```python
from build123d import *

# Parameters (mm, degrees)
F0_R     = 3.302
F0_R_2   = 16.51
F0_W     = 177.8
F0_H     = 77.7875
F1_DEPTH = 3.175


# Not quite as in the source:
# - ends of sketch curves that miss each other by under 0.0002 mm in the source are joined


with BuildPart() as f1:
    # F0 (on Front) → F1 (new body)
    with BuildSketch(Plane.XZ):
        with BuildLine():
            Line((-4.6405893252, -64.494198626), (72.172606051, -64.494198626))
            ThreePointArc((72.172606051, -64.494198626), (89.5045003647, -57.3150929397), (96.683606051, -39.983198626))
            Line((96.683606051, -39.983198626), (96.683606051, -30.0584486086))
            Line((96.683606051, -30.0584486086), (44.4719158113, 81.3992435336))
            Line((44.4719158113, 81.3992435336), (-29.9480052508, 81.3992435336))
            Line((-29.9480052508, 81.3992435336), (-35.9978974571, 50.6829957967))
            Line((-35.9978974571, 50.6829957967), (-19.4879078689, 50.6714224456))
            ThreePointArc((-19.4879078689, 50.6714224456), (-15.5812211009, 47.1637298884), (-13.9720730804, 42.1660573792))
            Line((-13.9720730804, 42.1660573792), (-5.4024819992, 38.3506346508))
            Line((-5.4024819992, 38.3506346508), (-2.9009456417, 36.1038269705))
            Line((-2.9009456417, 36.1038269705), (-2.3647786124, 27.9011076368))
            ThreePointArc((-2.3647786124, 27.9011076368), (3.4353485173, 23.5426794776), (4.3712937617, 16.3481414632))
            Line((4.3712937617, 16.3481414632), (4.2880776677, 1.0115236557))
            Line((4.2880776677, 1.0115236557), (-4.6405893252, -15.5276898319))
            Line((-4.6405893252, -15.5276898319), (-105.627393949, -15.5276898319))
            ThreePointArc((-105.627393949, -15.5276898319), (-130.1106483461, -40.010944229), (-105.627393949, -64.494198626))
            Line((-105.627393949, -64.494198626), (-4.6405893252, -64.494198626))
        make_face()
        with BuildLine():
            ThreePointArc((-105.627393949, -37.1117488528), (-103.5773532385, -37.9609035185), (-102.7281985728, -40.010944229))
            ThreePointArc((-102.7281985728, -40.010944229), (-103.5773532385, -42.0609849395), (-105.627393949, -42.9101396052))
            ThreePointArc((-105.627393949, -42.9101396052), (-107.6774346595, -42.0609849395), (-108.5265893252, -40.010944229))
            ThreePointArc((-108.5265893252, -40.010944229), (-107.6774346595, -37.9609035185), (-105.627393949, -37.1117488528))
        make_face(mode=Mode.SUBTRACT)
        with BuildLine():
            ThreePointArc((-4.6405893252, -54.334198626), (-2.3955252949, -55.2641345958), (-1.4655893252, -57.509198626))
            ThreePointArc((-1.4655893252, -57.509198626), (-2.3955252949, -59.7542626563), (-4.6405893252, -60.684198626))
            ThreePointArc((-4.6405893252, -60.684198626), (-6.8856533555, -59.7542626563), (-7.8155893252, -57.509198626))
            ThreePointArc((-7.8155893252, -57.509198626), (-6.8856533555, -55.2641345958), (-4.6405893252, -54.334198626))
        make_face(mode=Mode.SUBTRACT)
        with BuildLine():
            ThreePointArc((-4.6405893252, -19.282198626), (-2.3955252949, -20.2121345958), (-1.4655893252, -22.457198626))
            ThreePointArc((-1.4655893252, -22.457198626), (-2.3955252949, -24.7022626563), (-4.6405893252, -25.632198626))
            ThreePointArc((-4.6405893252, -25.632198626), (-6.8856533555, -24.7022626563), (-7.8155893252, -22.457198626))
            ThreePointArc((-7.8155893252, -22.457198626), (-6.8856533555, -20.2121345958), (-4.6405893252, -19.282198626))
        make_face(mode=Mode.SUBTRACT)
        with BuildLine():
            ThreePointArc((72.172606051, -37.0840032499), (74.2226467615, -37.9331579156), (75.0718014272, -39.983198626))
            ThreePointArc((75.0718014272, -39.983198626), (74.2226467615, -42.0332393365), (72.172606051, -42.8823940022))
            ThreePointArc((72.172606051, -42.8823940022), (70.1225653405, -42.0332393365), (69.2734106748, -39.983198626))
            ThreePointArc((69.2734106748, -39.983198626), (70.1225653405, -37.9331579156), (72.172606051, -37.0840032499))
        make_face(mode=Mode.SUBTRACT)
        with Locations((11.5432352797, 22.0017248669)):
            Circle(F0_R, mode=Mode.SUBTRACT)
        with Locations((-13.3156779021, 53.5307241817)):
            Circle(F0_R, mode=Mode.SUBTRACT)
        with Locations((11.6086210255, 54.3104703533)):
            Circle(F0_R_2, mode=Mode.SUBTRACT)
        with Locations((36.2912922688, 53.4994019413)):
            Circle(F0_R, mode=Mode.SUBTRACT)
        Polygon((72.172606051, -76.841138626), (72.172606051, -64.494198626), (-4.6405893252, -64.494198626), (-105.627393949, -64.494198626), (-105.627393949, -76.841138626), align=None)
        with Locations((-16.727393949, -115.734888626)):
            Rectangle(F0_W, F0_H)
        Polygon((72.172606051, -166.975578626), (72.172606051, -154.628638626), (-105.627393949, -154.628638626), (-105.627393949, -166.975578626), (-4.6405893252, -166.975578626), align=None)
        with BuildLine():
            ThreePointArc((96.683606051, -191.486578626), (89.5045003647, -174.1546843124), (72.172606051, -166.975578626))
            Line((72.172606051, -166.975578626), (-4.6405893252, -166.975578626))
            Line((-4.6405893252, -166.975578626), (-105.627393949, -166.975578626))
            ThreePointArc((-105.627393949, -166.975578626), (-130.1106483461, -191.4588330231), (-105.627393949, -215.9420874201))
            Line((-105.627393949, -215.9420874201), (-4.6405893252, -215.9420874201))
            Line((-4.6405893252, -215.9420874201), (4.2880776677, -232.4813009078))
            Line((4.2880776677, -232.4813009078), (4.3712937617, -247.8179187153))
            ThreePointArc((4.3712937617, -247.8179187153), (3.4353485173, -255.0124567297), (-2.3647786124, -259.3708848889))
            Line((-2.3647786124, -259.3708848889), (-2.9009456417, -267.5736042226))
            Line((-2.9009456417, -267.5736042226), (-5.4024819992, -269.8204119029))
            Line((-5.4024819992, -269.8204119029), (-13.9720735102, -273.635839865))
            ThreePointArc((-13.9720735102, -273.635839865), (-15.5812211009, -278.6335071405), (-19.487905219, -282.1411996959))
            Line((-19.487905219, -282.1411996959), (-35.9978974571, -282.1527730488))
            Line((-35.9978974571, -282.1527730488), (-29.9480052508, -312.8690207857))
            Line((-29.9480052508, -312.8690207857), (44.4719158113, -312.8690207857))
            Line((44.4719158113, -312.8690207857), (96.683606051, -201.4113286435))
            Line((96.683606051, -201.4113286435), (96.683606051, -191.486578626))
        make_face()
        with BuildLine():
            ThreePointArc((-105.627393949, -194.3580283993), (-107.6774346595, -193.5088737336), (-108.5265893252, -191.4588330231))
            ThreePointArc((-108.5265893252, -191.4588330231), (-107.6774346595, -189.4087923126), (-105.627393949, -188.5596376469))
            ThreePointArc((-105.627393949, -188.5596376469), (-103.5773532385, -189.4087923126), (-102.7281985728, -191.4588330231))
            ThreePointArc((-102.7281985728, -191.4588330231), (-103.5773532385, -193.5088737336), (-105.627393949, -194.3580283993))
        make_face(mode=Mode.SUBTRACT)
        with Locations((-13.3156779021, -285.0005014338)):
            Circle(F0_R, mode=Mode.SUBTRACT)
        with Locations((11.6086210255, -285.7802476054)):
            Circle(F0_R_2, mode=Mode.SUBTRACT)
        with Locations((36.2912922688, -284.9691791934)):
            Circle(F0_R, mode=Mode.SUBTRACT)
        with Locations((11.5432352796, -253.471502119)):
            Circle(F0_R, mode=Mode.SUBTRACT)
        with BuildLine():
            ThreePointArc((-1.4655893252, -209.012578626), (-2.3955252949, -211.2576426563), (-4.6405893252, -212.187578626))
            ThreePointArc((-4.6405893252, -212.187578626), (-6.8856533555, -211.2576426563), (-7.8155893252, -209.012578626))
            ThreePointArc((-7.8155893252, -209.012578626), (-6.8856533555, -206.7675145958), (-4.6405893252, -205.837578626))
            ThreePointArc((-4.6405893252, -205.837578626), (-2.3955252949, -206.7675145958), (-1.4655893252, -209.012578626))
        make_face(mode=Mode.SUBTRACT)
        with BuildLine():
            ThreePointArc((-1.4655893252, -173.960578626), (-2.3955252949, -176.2056426563), (-4.6405893252, -177.135578626))
            ThreePointArc((-4.6405893252, -177.135578626), (-6.8856533555, -176.2056426563), (-7.8155893252, -173.960578626))
            ThreePointArc((-7.8155893252, -173.960578626), (-6.8856533555, -171.7155145958), (-4.6405893252, -170.785578626))
            ThreePointArc((-4.6405893252, -170.785578626), (-2.3955252949, -171.7155145958), (-1.4655893252, -173.960578626))
        make_face(mode=Mode.SUBTRACT)
        with BuildLine():
            ThreePointArc((72.172606051, -194.3857740022), (70.1225653405, -193.5366193365), (69.2734106748, -191.486578626))
            ThreePointArc((69.2734106748, -191.486578626), (70.1225653405, -189.4365379156), (72.172606051, -188.5873832499))
            ThreePointArc((72.172606051, -188.5873832499), (74.2226467615, -189.4365379156), (75.0718014272, -191.486578626))
            ThreePointArc((75.0718014272, -191.486578626), (74.2226467615, -193.5366193365), (72.172606051, -194.3857740022))
        make_face(mode=Mode.SUBTRACT)
    extrude(amount=F1_DEPTH)


solid = f1.part
```
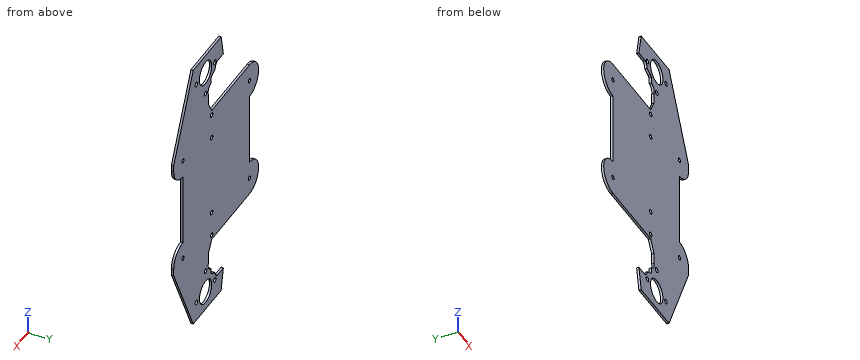
CAD build for the part. Positions are in the model's coordinates, mm. Give positions to 0.01 mm unless a question says otherwise; leave off trailing zeros. Order: outer loops, then holes, each group sorted by start corner. A loop starts at its lowest first (then second) coordinate and runs counter-clockwise, first axis right, second up.
(1) Drill centre lines: L1, parallel to Z at x = -106, y = -1.2; L2, parallel to Z at x = -21, y = -2.2; L3, parallel to X at y = -0.5, z = -192.5. Where is each one in solid material? Low to high.
(2) Saw through at B-B, the plane z = -99. Give the cut face in (x, y) (3 decimals), then the cut area to 3 significant figures.
(3) Saw through at D-D, the plane z = -243.5. Give the cut face in (x, y) (3 decimals).
(4) Saw through at C-C, the plane y = -1.05. State how many separate pieces and enclosed holes the cut face has, then the cut area to 3 significant figures.
(5) Saw through at A-A, the plane x = 22. Give the cut face in (y, z) (3 decimals), then the cut area to 3 significant figures.
(6) Flat gauge pins, fed straight in: pin 1 (5.5 mm diameter, centred on x = -13.32, z = 53.53, fed in from -Y); pin 2 (1 mm diameter, centred on x = -92.5, y = -0.5, fed in from +Z); pin 3 (1 mm diameter, centred on x = -55, y = -1.5, fed in from -Z). Where does each tip first touch, or does it go through?
Results found:
1. L1: z = -215.94 to -194.33, -188.58 to -166.98, -64.49 to -42.89, -37.14 to -15.53
1. L2: z = -312.87 to -282.14, -215.94 to -15.53, 50.67 to 81.4
1. L3: x = -130.09 to -108.33, -102.92 to 69.46, 74.89 to 96.68
2. outline: (-105.627, -3.175) - (72.173, -3.175) - (72.173, 0) - (-105.627, 0) - close
2. area: 565 mm2
3. outline: (4.348, -3.175) - (76.967, -3.175) - (76.967, 0) - (4.348, 0) - close
4. separate pieces: 1
4. enclosed holes: 16
4. area: 52,700 mm2
5. outline: (-3.175, -312.869) - (0, -312.869) - (0, -298.61) - (-3.175, -298.61) - close; (-3.175, -272.951) - (0, -272.951) - (0, 41.481) - (-3.175, 41.481) - close; (-3.175, 67.14) - (0, 67.14) - (0, 81.399) - (-3.175, 81.399) - close
5. area: 1,090 mm2
6. pin 1: passes through
6. pin 2: stops at z = -15.53
6. pin 3: stops at z = -215.94
